from build123d import *

# Parameters (mm, degrees)
SKETCH1_W           = 55
SKETCH1_H           = 62
SKETCH1_W_2         = 25
SKETCH1_H_2         = 45
BOSS_EXTRUDE1_DEPTH = 4
SKETCH2_W           = 7.5
SKETCH2_H           = 8
SKETCH2_R           = 1.5
BOSS_EXTRUDE2_DEPTH = 4


with BuildPart() as part:
    # Sketch1 → Boss-Extrude1 (new body)
    with BuildSketch(Plane(origin=(0, 0, 0), x_dir=(1, 0, 0), z_dir=(0, 1, 0))):
        Rectangle(SKETCH1_W, SKETCH1_H)
        Rectangle(SKETCH1_W_2, SKETCH1_H_2, mode=Mode.SUBTRACT)
    extrude(amount=BOSS_EXTRUDE1_DEPTH)

    # Sketch2 → Boss-Extrude2 (add)
    # profile 1 of 2: a face of its own
    with BuildSketch(Plane.XY.offset(31)):
        with Locations((-23.75, 8)):
            Rectangle(SKETCH2_W, SKETCH2_H)
        with Locations((-23.75, 8)):
            Circle(SKETCH2_R, mode=Mode.SUBTRACT)
    # profile 2 of 2: a face of its own
    with BuildSketch(Plane.XY.offset(31)):
        with Locations((23.75, 8)):
            Rectangle(SKETCH2_W, SKETCH2_H)
        with Locations(Location((23.75, 8, 0), (0, 0, 180))):
            Circle(SKETCH2_R, mode=Mode.SUBTRACT)
    boss_extrude2 = extrude(amount=-BOSS_EXTRUDE2_DEPTH)

    # Mirror1: Boss-Extrude2 across plane
    add(boss_extrude2.mirror(Plane.XY))


solid = part.part
Part model, mm, in its own coordinate system. A direction names the side the tool comes from. Coordinates: 2 decimals unless noted, no trailing zeros. Loops run counter-clockwise (first coordinate to the right, second up) from the corner with the lowest first, then second, coordinate; pieces in that order, holes last. Notation, with made-up numbers: (62, 86) - (109, 86) arc R6 cw to (109, 91) - close; hole circle Ø6 at (-16, 1.25). An arc over 180 degrees is marked (long way). Write each question's results on one line, items separated by ' | '. Start each with the question number.
Q1. Probe line 1 along Z through (x, y) = (-10, 3); line 2 along Z through (x, y) = (22, 8.25); line 3 along X through (y, z) = (3, 14.5). List the from-to ranges inside material, lowest first.
Q2. Slice it at B-B on z = -20.5. Give the cut face in (x, y).
Q3. Which spindle directions (+Z, -Z, +X, -X, +Y, -Y) get a long thin tool onto all of the face, cutting with end or side? Do faces 5 (the flat face through (22, 8, 27)), 6 (the flat face through (-20, 8, -29)), 7 (the flat face through (-13, 0, 0)), 8 (the flat face through (12.5, 2, 0)). Say none if no direction does.
Q4. Drop flat-ended pins along their axis: pin 1 Ø1.8 at (x, y) = (-23.75, 8) entering from +Z; pin 2 Ø1.5 at (x, z) = (-9, 24) entering from +Y. Give the stop position or say it passes through.
Q5. Slice it at D-D on x = -11.5. Give the cut face in (y, z), and give its area (3 significant figures).
Q6. Two-plate mould, pull along X, no slides. Class faces 1 (the flat face through (-20, 8, 29)), 2 (the flat face through (-27.5, 3, 0)), 3 (the cylindrical face through (24.94, 8.91, 29.03)), 4 (the flat face through (22, 8, -27)): +X half, -X half, draft (parallel to the pull), parting line (faces both ways), or undercut.
Q7. Slice it at A-A on x = -23.75. Give the cut face in (y, z), and give its area (3 significant figures).
Q8. Slice it at C-C on y = 8. Give the number of separate pieces and of enclosed holes in the cut face, and give its area (3 significant figures).
Answer:
1) line 1: z = -31 to -22.5, 22.5 to 31 | line 2: z = -31 to -27, 27 to 31 | line 3: x = -27.5 to -12.5, 12.5 to 27.5
2) outline: (-27.5, 0) - (-12.5, 0) - (-12.5, 4) - (-27.5, 4) - close; (12.5, 0) - (27.5, 0) - (27.5, 4) - (12.5, 4) - close
3) face 5: +X, -X, +Y | face 6: +Z, -Z, +Y | face 7: +Z, -Z, +X, -X, -Y | face 8: +Y, -Y
4) pin 1: passes through | pin 2: stops at y = 4
5) outline: (0, -31) - (4, -31) - (4, -22.5) - (0, -22.5) - close; (0, 22.5) - (4, 22.5) - (4, 31) - (0, 31) - close | area: 68.0 mm2
6) face 1: undercut | face 2: -X half | face 3: undercut | face 4: draft
7) outline: (0, -31) - (6.5, -31) - (6.5, -27) - (4, -27) - (4, 27) - (6.5, 27) - (6.5, 31) - (0, 31) - close; (9.5, -31) - (12, -31) - (12, -27) - (9.5, -27) - close; (9.5, 27) - (12, 27) - (12, 31) - (9.5, 31) - close | area: 288 mm2
8) separate pieces: 8 | enclosed holes: 0 | area: 72.0 mm2
